```python
from build123d import *

# Parameters (mm, degrees)
F0_R     = 25.3
F1_DEPTH = 3.3
F3_DEPTH = 12.5
F4_R     = 5.1
F5_DEPTH = 15.801


with BuildPart() as f1:
    # F0 (on Top) → F1 (new body)
    with BuildSketch(Plane.XY):
        Circle(F0_R)
    extrude(amount=F1_DEPTH)

    # F2 (on face) → F3 (join)
    with BuildSketch(Plane.XY.offset(3.3)):
        with BuildLine():
            ThreePointArc((19.908332, -10.483718), (21.842475, -5.399655), (22.5, 0))
            ThreePointArc((22.5, 0), (21.842475, 5.399655), (19.908332, 10.483718))
            ThreePointArc((19.908332, 10.483718), (19.485572, 11.25), (19.033332, 11.999262))
            ThreePointArc((19.033332, 11.999262), (11.25, 19.485572), (0.875, 22.48298))
            ThreePointArc((0.875, 22.48298), (0, 22.5), (-0.875, 22.48298))
            ThreePointArc((-0.875, 22.48298), (-11.25, 19.485572), (-19.033332, 11.999262))
            ThreePointArc((-19.033332, 11.999262), (-19.485572, 11.25), (-19.908332, 10.483718))
            ThreePointArc((-19.908332, 10.483718), (-22.5, 0), (-19.908332, -10.483718))
            ThreePointArc((-19.908332, -10.483718), (-19.485572, -11.25), (-19.033332, -11.999262))
            ThreePointArc((-19.033332, -11.999262), (-11.25, -19.485572), (-0.875, -22.48298))
            ThreePointArc((-0.875, -22.48298), (0, -22.5), (0.875, -22.48298))
            ThreePointArc((0.875, -22.48298), (11.25, -19.485572), (19.033332, -11.999262))
            ThreePointArc((19.033332, -11.999262), (19.485572, -11.25), (19.908332, -10.483718))
        make_face()
        with BuildLine():
            ThreePointArc((19.033332, 11.999262), (19.485572, 11.25), (19.908332, 10.483718))
            Line((19.908332, 10.483718), (20.702494, 10.942228))
            Line((20.702494, 10.942228), (19.827494, 12.457772))
            Line((19.827494, 12.457772), (19.033332, 11.999262))
        make_face()
        with BuildLine():
            Line((20.702494, -10.942228), (19.908332, -10.483718))
            ThreePointArc((19.908332, -10.483718), (19.485572, -11.25), (19.033332, -11.999262))
            Line((19.033332, -11.999262), (19.827494, -12.457772))
            Line((19.827494, -12.457772), (20.702494, -10.942228))
        make_face()
        with BuildLine():
            ThreePointArc((-0.875, 22.48298), (0, 22.5), (0.875, 22.48298))
            Line((0.875, 22.48298), (0.875, 23.4))
            Line((0.875, 23.4), (-0.875, 23.4))
            Line((-0.875, 23.4), (-0.875, 22.48298))
        make_face()
        with BuildLine():
            Line((0.875, -23.4), (0.875, -22.48298))
            ThreePointArc((0.875, -22.48298), (0, -22.5), (-0.875, -22.48298))
            Line((-0.875, -22.48298), (-0.875, -23.4))
            Line((-0.875, -23.4), (0.875, -23.4))
        make_face()
        with BuildLine():
            ThreePointArc((-19.908332, 10.483718), (-19.485572, 11.25), (-19.033332, 11.999262))
            Line((-19.033332, 11.999262), (-19.827494, 12.457772))
            Line((-19.827494, 12.457772), (-20.702494, 10.942228))
            Line((-20.702494, 10.942228), (-19.908332, 10.483718))
        make_face()
        with BuildLine():
            Line((-19.827494, -12.457772), (-19.033332, -11.999262))
            ThreePointArc((-19.033332, -11.999262), (-19.485572, -11.25), (-19.908332, -10.483718))
            Line((-19.908332, -10.483718), (-20.702494, -10.942228))
            Line((-20.702494, -10.942228), (-19.827494, -12.457772))
        make_face()
    extrude(amount=F3_DEPTH)

    # F4 (on face) → F5 (cut, through all)
    with BuildSketch(Plane.XY.offset(15.8)):
        Circle(F4_R)
    extrude(amount=-F5_DEPTH, mode=Mode.SUBTRACT)


solid = f1.part
```
Design review of the part built by this model. Coordinates are the model's own, in mm. A direction names the side the tool comes from. Coordinates: 2 decimals unless noted, no trailing zeros. Order: outer loops, then holes, each group sorted by start corner. A loop starts at its lowest first (then second) coordinate and runs counter-clockwise, first axis right, second up.
1) Take a section at B-B, the plane z = 13.5. Give the boundary of the cut face in (x, y) (1 decimal).
2) Take a section at A-A, the plane x = 0. Give the boundary of the cut face in (y, z), and give its area (3 significant figures).
3) Mouldability with a two-part tool opening along X and no side actions: class faces 1 (the cylindrical face through (2.4, -4.5, 8)), 2 (the cylindrical face through (-5.48, -24.7, 1.63)), 3 (the flat face through (-20.26, 11.71, 9.46)) as +X half, -X half, draft (parallel to the pull), parting line (faces both ways), or undercut.
4) For faces 4 (the flat face through (-20.27, -11.69, 9.46)), 5 (the flat face through (0, -23.4, 9)), 6 (the flat face through (0, 23.4, 9)), list the 3-axis set-ups (+Z, -Z, +X, -X, +Y, -Y) from which the entire face can be reached by the end or side of a thin tool; tool diameter is ignored.
5) Wall thickness on line 1 along Y through (x, z) = (0, 11.25); line 2 along Y through (x, z) = (-2.5, 4.5); line 3 along X through (y, z) = (4.5, 2.75): over which ranges is each line inside the solid? List them lowest first.
6) Take a section at D-D, the plane x = -10. Give the boundary of the cut face in (y, z), and give its area (3 significant figures).
7) Clearance check with flat-ended pins moving along their axes: pin 1 (2 mm diameter, centred on x = 17.5, z = 9, fed in from +Y); pin 2 (0.5 mm diameter, centred on y = -23, z = 11, fed in from +X) (3 decimals); pin 3 (0.5 mm diameter, centred on x = 0, z = 10, fed in from -Y). State where each tip first meets the part, or that it passes through.
8) Take a section at C-C, the plane y = 4. Give the boundary of the cut face in (x, z).
Returned:
1. outline: (-20.7, -10.9) - (-19.8, -12.5) - (-19, -12) arc R22.5 ccw to (-0.9, -22.5) - (-0.9, -23.4) - (0.9, -23.4) - (0.9, -22.5) arc R22.5 ccw to (19, -12) - (19.8, -12.5) - (20.7, -10.9) - (19.9, -10.5) arc R22.5 ccw to (22.5, 0) arc R22.5 ccw to (19.9, 10.5) - (20.7, 10.9) - (19.8, 12.5) - (19, 12) arc R22.5 ccw to (0.9, 22.5) - (0.9, 23.4) - (-0.9, 23.4) - (-0.9, 22.5) arc R22.5 ccw to (-19, 12) - (-19.8, 12.5) - (-20.7, 10.9) - (-19.9, 10.5) arc R22.5 ccw to (-19.9, -10.5) - close; hole circle Ø10.2 at (0, 0)
2. outline: (-25.3, 0) - (-5.1, 0) - (-5.1, 15.8) - (-23.4, 15.8) - (-23.4, 3.3) - (-25.3, 3.3) - close; (5.1, 0) - (25.3, 0) - (25.3, 3.3) - (23.4, 3.3) - (23.4, 15.8) - (5.1, 15.8) - close
2. area: 591 mm2
3. face 1: undercut
3. face 2: parting line
3. face 3: -X half
4. face 4: +Z, -X, -Y
4. face 5: +Z, +X, -X, -Y
4. face 6: +Z, +X, -X, +Y
5. line 1: y = -23.4 to -5.1, 5.1 to 23.4
5. line 2: y = -22.36 to -4.45, 4.45 to 22.36
5. line 3: x = -24.9 to -2.4, 2.4 to 24.9
6. outline: (-23.24, 0) - (23.24, 0) - (23.24, 3.3) - (20.16, 3.3) - (20.16, 15.8) - (-20.16, 15.8) - (-20.16, 3.3) - (-23.24, 3.3) - close
6. area: 657 mm2
7. pin 1: stops at y = 15.3
7. pin 2: stops at x = 0.875
7. pin 3: stops at y = -23.4
8. outline: (-24.98, 0) - (-3.16, 0) - (-3.16, 15.8) - (-22.14, 15.8) - (-22.14, 3.3) - (-24.98, 3.3) - close; (3.16, 0) - (24.98, 0) - (24.98, 3.3) - (22.14, 3.3) - (22.14, 15.8) - (3.16, 15.8) - close
